Check sheet for the modelled part. Datum: model origin and axes. Units: mm. Give positions to 0.01 mm unless a question says otherwise; leave off trailing zeros. Order: outer loops, then holes, each group sorted by start corner. A loop starts at its lowest first (then second) coordinate and runs counter-clockwise, first axis right, second up.
```python
from build123d import *

# Parameters (mm, degrees)
SKETCH2_W           = 49
SKETCH2_H           = 71.5
BOSS_EXTRUDE1_DEPTH = 2
SKETCH2_6_R         = 1
SKETCH2_6_R_2       = 7.5
SKETCH2_6_R_3       = 2
CUT_EXTRUDE2_DEPTH  = 10
FILLET1_R           = 5


with BuildPart() as part:
    # Sketch2 → Boss-Extrude1 (new body)
    with BuildSketch(Plane(origin=(0, 0, 0), x_dir=(1, 0, 0), z_dir=(0, 1, 0))):
        Rectangle(SKETCH2_W, SKETCH2_H)
    extrude(amount=BOSS_EXTRUDE1_DEPTH)

    # Sketch2<6> → Cut-Extrude2 (cut)
    with BuildSketch(Plane(origin=(0, 0, 0), x_dir=(1, 0, 0), z_dir=(0, 1, 0))):
        with Locations((-22, 30.5)):
            Circle(SKETCH2_6_R)
        with Locations((22, 30.5)):
            Circle(SKETCH2_6_R)
        with Locations((-22, -30.5)):
            Circle(SKETCH2_6_R)
        with Locations((22, -30.5)):
            Circle(SKETCH2_6_R)
        Circle(SKETCH2_6_R_2)
        with Locations((11.313708499, 11.313708499)):
            Circle(SKETCH2_6_R_3)
        with Locations((11.313708499, -11.313708499)):
            Circle(SKETCH2_6_R_3)
        with Locations((-11.313708499, -11.313708499)):
            Circle(SKETCH2_6_R_3)
        with Locations((-11.313708499, 11.313708499)):
            Circle(SKETCH2_6_R_3)
    extrude(amount=CUT_EXTRUDE2_DEPTH, mode=Mode.SUBTRACT)

    # Fillet1
    fillet1_edges = [part.edges().sort_by_distance(p)[0] for p in [
        (-24.5, 1, -35.75),
        (-24.5, 1, 35.75),
        (24.5, 1, 35.75),
        (24.5, 1, -35.75),
    ]]
    fillet(fillet1_edges, radius=FILLET1_R)


solid = part.part
```
(1) Sectioned sample at D-D (x = 22). Enter the section's corners in (y, z).
(2) Sectioned sample at A-A (z = 0). Enter the section's corners in (x, y), plus the area to 3 significant figures.
(3) Thickness scan on L1, parallel to X at y = 0.55, z = -30.5; L2, parallel to X at y = 0.5, z = -11.5; L3, parallel to Z at x = -22, y = 1.35. Record the ranges inside material, lowest first.
(4) Sectioned sample at C-C (y = 1.6). Count the separate pieces of the cut face and the enclosed holes in it, plus the area to 3 significant figures.
(5) Sectioned sample at B-B (x = 0). Enter the section's corners in (y, z), plus the area to 3 significant figures.
(6) Release check for a two-part mould opening along X. For faces 1 (the face through (-24.5, 1, 0)), 2 (the face through (0, 1, 35.75)), 3 (the face through (-11.75, 0.99, -9.36)) record: released by +X, released by -X, zero draft, split by the parting line, or undercut.
Values follow:
1. outline: (0, -35.08) - (2, -35.08) - (2, -31.5) - (0, -31.5) - close; (0, -29.5) - (2, -29.5) - (2, 29.5) - (0, 29.5) - close; (0, 31.5) - (2, 31.5) - (2, 35.08) - (0, 35.08) - close
2. outline: (-24.5, 0) - (-7.5, 0) - (-7.5, 2) - (-24.5, 2) - close; (7.5, 0) - (24.5, 0) - (24.5, 2) - (7.5, 2) - close
2. area: 68.0 mm2
3. L1: x = -24.5 to -23, -21 to 21, 23 to 24.5
3. L2: x = -24.5 to -13.31, -9.32 to 9.32, 13.31 to 24.5
3. L3: z = -35.08 to -31.5, -29.5 to 29.5, 31.5 to 35.08
4. separate pieces: 1
4. enclosed holes: 9
4. area: 3,240 mm2
5. outline: (0, -35.75) - (2, -35.75) - (2, -7.5) - (0, -7.5) - close; (0, 7.5) - (2, 7.5) - (2, 35.75) - (0, 35.75) - close
5. area: 113 mm2
6. face 1: released by -X
6. face 2: zero draft
6. face 3: undercut
